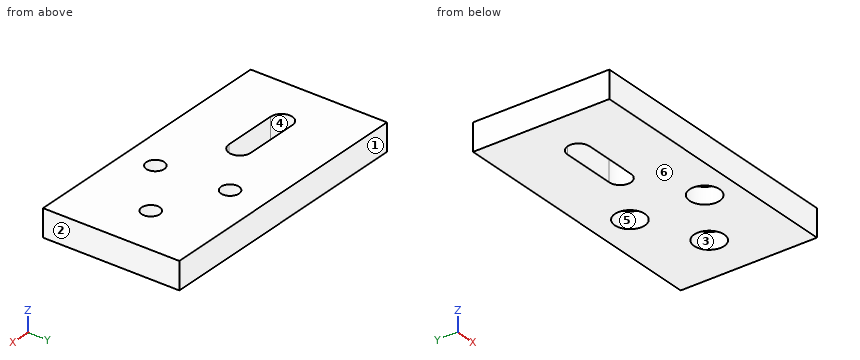
Autodesk Fusion 360 part; units mm, degrees
sketch "Sketch1" plane through (0, 0, 0) normal (0, 0, 1) x (1, 0, 0)
  line L0 (0, 0) -> (100, 0)
  line L1 (100, 0) -> (100, 50)
  line L2 (100, 50) -> (0, 50)
  line L3 (0, 50) -> (0, 0)
  circle A0 centre (82.132, 25.9392) radius 5.5
  circle A1 centre (60.7017, 11.2509) radius 5.5
  circle A2 centre (58.6964, 37.1542) radius 3
  line L4 (18, 29) -> (38, 29)
  line L5 (18, 21) -> (38, 21)
  arc A3 (18, 29) -> (18, 21) centre (18, 25) ccw
  arc A4 (38, 21) -> (38, 29) centre (38, 25) ccw
  circle A5 centre (58.6964, 37.1542) radius 5.5
  circle A6 centre (60.7017, 11.2509) radius 3.3
  circle A7 centre (82.132, 25.9392) radius 3.3
  dimension "d24" = 11
  dimension "d25" = 11
  dimension "d26" = 6.6
  dimension "d27" = 11
  dimension "d28" = 6.6
sketch "Sketch2" plane through (0, 0, 0) normal (0, 0, 1) x (1, 0, 0)
extrude "Extrude1" add sketch "Sketch1" along normal blind 10 contours L0 L1 L2 L3 | A0 | A1 | A2 | A5 | A6 | A7
hole "Hole1" at (58.6964, 37.1542, 0) at (60.7017, 11.2509, 0) at (82.132, 25.9392, 0) direction (0, 0, 1) diameter 6.6 depth 20 tip angle 118 counterbore diameter 11 counterbore depth 6
Read the model definition and answer for the solid it produces. Units are mm, in the model's axes. Face numbers are marked on the shaded views. A direction names the side the tool comes from. Coordinates: 2 decimals unless noted, no trailing zeros. Loops run counter-clockwise (first coordinate to the right, second up) from the corner with the lowest first, then second, coordinate; pieces in that order, holes last.
Q1. Consider probe 1 along X at (y, z) = (28.5, 1.5); probe 2 along X at (y, z) = (11.5, 7); probe 3 along X at (y, z) = (24, 6.25). Determine where each line is inside the solid, lowest interval first.
Q2. The part is cut by section B-B on z = 7. Write down the section's boundary in (x, y), and give its area (3 significant figures).
Q3. The part is cut by section C-C on y = 10. Write down the section's boundary in (x, z).
Q4. The part is cut by section A-A on y = 25. Write down the section's boundary in (x, z), and give its area (3 significant figures).
Q5. The mould has two halves that part along X. Classify the marked faces 1, 2 and 3: +X half, -X half, draft (parallel to the pull), parting line (faces both ways), or undercut.
Q6. Which of the six approach directions +Z, -Z, +X, -X, +Y, -Y give full straight-line access (tool end or side, diameter ignored) to the marked faces 4, 5 and 6?
Q7. Each of these flat-tipped pins is pushed along its axis until it touches: pin 1 Ø5 at (y, z) = (39, 3.5) entering from -X; pin 2 Ø10.5 at (x, y) = (58.7, 37.15) entering from -Z; pin 3 Ø6.5 at (x, y) = (82.13, 25.94) entering from -Z (3 decimals). Where does it stop, or does it pass through?
Results below:
1. probe 1: x = 0 to 16.06, 39.94 to 77.26, 87 to 100
1. probe 2: x = 0 to 57.41, 63.99 to 100
1. probe 3: x = 0 to 14.13, 41.87 to 79.46, 84.8 to 100
2. outline: (0, 0) - (100, 0) - (100, 50) - (0, 50) - close; hole (18, 21) - (38, 21) arc R4 ccw to (38, 29) - (18, 29) arc R4 ccw to start; hole circle Ø6.6 at (58.7, 37.15); hole circle Ø6.6 at (60.7, 11.25); hole circle Ø6.6 at (82.13, 25.94)
2. area: 4,690 mm2
3. outline: (0, 0) - (55.35, 0) - (55.35, 6) - (57.65, 6) - (57.65, 10) - (0, 10) - close; (63.76, 6) - (66.06, 6) - (66.06, 0) - (100, 0) - (100, 10) - (63.76, 10) - close
4. outline: (0, 0) - (14, 0) - (14, 10) - (0, 10) - close; (42, 0) - (76.71, 0) - (76.71, 6) - (78.97, 6) - (78.97, 10) - (42, 10) - close; (85.3, 6) - (87.55, 6) - (87.55, 0) - (100, 0) - (100, 10) - (85.3, 10) - close
4. area: 630 mm2
5. face 1: draft
5. face 2: +X half
5. face 3: undercut
6. face 4: +Z, -Z
6. face 5: -Z
6. face 6: -Z, +X, -X, +Y, -Y
7. pin 1: stops at x = 0
7. pin 2: stops at z = 6
7. pin 3: passes through
